Geometry: final body of the model. Coordinates: model frame, mm. A direction names the side the tool comes from. Give positions to 0.01 mm unless a question says otherwise; leave off trailing zeros. Write each loop counter-clockwise with the first axis right and the second up, starting at its lowest first coordinate (ties: lowest second). Pieces come first, ordered by that corner, then holes. Notation, with made-up numbers: (21, 42.5) -> (51, 42.5) arc R17 ccw to (51, 66.5) -> close; hole circle Ø9 at (29.5, 82.25). An arc over 180 degrees is marked (long way). Answer as a JSON object with one key per item and string values. Group by question number.
(1) Section query A-A on y = 48.5. Output: boundary loops of the cut face in (x, z).
(2) Section query B-B on x = 8. Output: boundary loops of the cut face in (y, z).
(3) Material intervals for probe 1 along Y at (x, z) = (25, 3.65); probe 2 along X at (y, z) = (43, 0.85); probe 3 along X at (y, z) = (48.5, 2.65), sorted ascending.
(4) Set-up query: faces 4 (the face through (73, 32, 2)), 5 (the face through (49, 31, 5)), 6 (the face through (92, 56, 2)). Return all of +Z, -Z, +X, -X, +Y, -Y with unobstructed straight access to the full face (end or side cutting, diameter ignored); none if empty.
(5) Draft query along Y for faces 1 (the face through (49, 31, 0)), 2 (the face through (60, 15, 2)), 3 (the face through (8, 46, 2)). Return one class per face: +Y half, -Y half, draft (parallel to the pull), parting line (faces both ways), or undercut.
(6) Contact query for flat-ended pins moving along their axis: pin 1 Ø2 at (x, z) = (79, 2) entering from +Y; pin 2 Ø1 at (x, z) = (79, 1) entering from -Y. Output: stop coordinate, or through.
(7) Section query D-D on y = 6.5. Output: boundary loops of the cut face in (x, z), plus the area to 3 significant figures.
(8) Section query C-C on x = 25. Output: boundary loops of the cut face in (y, z).
from build123d import *

# Parameters (mm, degrees)
ESQUISSE1_R        = 1.5
ESQUISSE1_W        = 5
ESQUISSE1_H        = 10
BOSS_EXTRU_1_DEPTH = 5


with BuildPart() as part:
    # Esquisse1 → Boss.-Extru.1 (new body)
    with BuildSketch(Plane.XY):
        with BuildLine():
            Line((0, 0), (31.277186767, 0))
            ThreePointArc((31.277186767, 0), (60, 15), (88.722813233, 0))
            Line((88.722813233, 0), (100, 0))
            Line((100, 0), (100, 61))
            Line((100, 61), (84, 61))
            Line((84, 61), (84, 39))
            Line((84, 39), (83, 39))
            Line((83, 39), (83, 32))
            Line((83, 32), (63, 32))
            Line((63, 32), (63, 41))
            Line((63, 41), (44.050031289, 41))
            Line((44.050031289, 41), (44.050031289, 61))
            Line((44.050031289, 61), (0, 61))
            Line((0, 61), (0, 0))
        make_face()
        with Locations((15, 6.5)):
            Circle(ESQUISSE1_R, mode=Mode.SUBTRACT)
        with Locations((25, 6.5)):
            Circle(ESQUISSE1_R, mode=Mode.SUBTRACT)
        with Locations(Location((25, 54.5, 0), (0, 0, 180))):
            Circle(ESQUISSE1_R, mode=Mode.SUBTRACT)
        with Locations(Location((15, 54.5, 0), (0, 0, 180))):
            Circle(ESQUISSE1_R, mode=Mode.SUBTRACT)
        with Locations((90, 20)):
            Circle(ESQUISSE1_R, mode=Mode.SUBTRACT)
        Polygon((10, 51), (19, 51), (19, 57), (21, 57), (21, 51), (30, 51), (30, 10), (21, 10), (21, 4), (19, 4), (19, 10), (10, 10), (10, 31), (5, 31), (5, 41), (10, 41), (10, 46), (5, 46), (5, 56), (10, 56), align=None, mode=Mode.SUBTRACT)
        with Locations((92.5, 51)):
            Rectangle(ESQUISSE1_W, ESQUISSE1_H, mode=Mode.SUBTRACT)
        with Locations((92.5, 36)):
            Rectangle(ESQUISSE1_W, ESQUISSE1_H, mode=Mode.SUBTRACT)
    extrude(amount=BOSS_EXTRU_1_DEPTH)


solid = part.part
Answer list:
{
 "1": {"outline": "(0, 0) -> (5, 0) -> (5, 5) -> (0, 5) -> close; (30, 0) -> (44.05, 0) -> (44.05, 5) -> (30, 5) -> close; (84, 0) -> (90, 0) -> (90, 5) -> (84, 5) -> close; (95, 0) -> (100, 0) -> (100, 5) -> (95, 5) -> close"},
 "2": {"outline": "(0, 0) -> (31, 0) -> (31, 5) -> (0, 5) -> close; (41, 0) -> (46, 0) -> (46, 5) -> (41, 5) -> close; (56, 0) -> (61, 0) -> (61, 5) -> (56, 5) -> close"},
 "3": {"probe 1": "0 to 5, 8 to 10, 51 to 53, 56 to 61", "probe 2": "0 to 10, 30 to 44.05, 84 to 100", "probe 3": "0 to 5, 30 to 44.05, 84 to 90, 95 to 100"},
 "4": {"face 4": "+Z, -Z, +Y", "face 5": "+Z, +X, -X, +Y, -Y", "face 6": "+Z, -Z"},
 "5": {"face 1": "draft", "face 2": "-Y half", "face 3": "undercut"},
 "6": {"pin 1": "y = 32", "pin 2": "y = 9.06"},
 "7": {"outline": "(0, 0) -> (13.5, 0) -> (13.5, 5) -> (0, 5) -> close; (16.5, 0) -> (19, 0) -> (19, 5) -> (16.5, 5) -> close; (21, 0) -> (23.5, 0) -> (23.5, 5) -> (21, 5) -> close; (26.5, 0) -> (37.14, 0) -> (37.14, 5) -> (26.5, 5) -> close; (82.86, 0) -> (100, 0) -> (100, 5) -> (82.86, 5) -> close", "area": "231 mm2"},
 "8": {"outline": "(0, 0) -> (5, 0) -> (5, 5) -> (0, 5) -> close; (8, 0) -> (10, 0) -> (10, 5) -> (8, 5) -> close; (51, 0) -> (53, 0) -> (53, 5) -> (51, 5) -> close; (56, 0) -> (61, 0) -> (61, 5) -> (56, 5) -> close"}
}
